```python
from build123d import *

# Parameters (mm, degrees)
SKETCH1_W           = 200
SKETCH1_H           = 200
BOSS_EXTRUDE1_DEPTH = 5
SKETCH3_R           = 2.5
CUT_EXTRUDE2_DEPTH  = 5
CUT_EXTRUDE4_DEPTH  = 200
CHAMFER1_SIZE       = 50
SKETCH5_R           = 2.5
CUT_EXTRUDE5_DEPTH  = 10


with BuildPart() as part:
    # Sketch1 → Boss-Extrude1 (new body)
    with BuildSketch(Plane(origin=(0, 0, 0), x_dir=(1, 0, 0), z_dir=(0, 1, 0))):
        with Locations((100, 100)):
            Rectangle(SKETCH1_W, SKETCH1_H)
    extrude(amount=BOSS_EXTRUDE1_DEPTH)

    # Sketch3 → Cut-Extrude2 (cut)
    with BuildSketch(Plane(origin=(0, 5, 0), x_dir=(1, 0, 0), z_dir=(0, 1, 0))):
        with Locations(Location((180, 62.426406871, 0), (0, 0, 270))):
            Circle(SKETCH3_R)
        with Locations(Location((90.710678119, 48.284271247, 0), (0, 0, 90))):
            Circle(SKETCH3_R)
        with Locations(Location((109.289321881, 48.284271247, 0), (0, 0, 270))):
            Circle(SKETCH3_R)
        with Locations(Location((62.426406871, 20, 0), (0, 0, 90))):
            Circle(SKETCH3_R)
        with Locations(Location((137.573593129, 20, 0), (0, 0, 270))):
            Circle(SKETCH3_R)
        with Locations(Location((20, 62.426406871, 0), (0, 0, 270))):
            Circle(SKETCH3_R)
        with Locations(Location((48.284271247, 90.710678119, 0), (0, 0, 270))):
            Circle(SKETCH3_R)
        with Locations(Location((20, 137.573593129, 0), (0, 0, 90))):
            Circle(SKETCH3_R)
        with Locations(Location((48.284271247, 109.289321881, 0), (0, 0, 90))):
            Circle(SKETCH3_R)
        with Locations(Location((62.426406871, 180, 0), (0, 0, 270))):
            Circle(SKETCH3_R)
        with Locations(Location((90.710678119, 151.715728753, 0), (0, 0, 270))):
            Circle(SKETCH3_R)
        with Locations(Location((109.289321881, 151.715728753, 0), (0, 0, 90))):
            Circle(SKETCH3_R)
        with Locations(Location((137.573593129, 180, 0), (0, 0, 90))):
            Circle(SKETCH3_R)
        with Locations(Location((180, 137.573593129, 0), (0, 0, 270))):
            Circle(SKETCH3_R)
        with Locations(Location((151.715728753, 109.289321881, 0), (0, 0, 270))):
            Circle(SKETCH3_R)
        with Locations(Location((151.715728753, 90.710678119, 0), (0, 0, 90))):
            Circle(SKETCH3_R)
    extrude(amount=-CUT_EXTRUDE2_DEPTH, mode=Mode.SUBTRACT)

    # Sketch4 → Cut-Extrude4 (cut)
    with BuildSketch(Plane(origin=(0, 5, 0), x_dir=(1, 0, 0), z_dir=(0, 1, 0))):
        Polygon((114.142135624, 121.213203436), (121.213203436, 114.142135624), (124.748737342, 117.67766953), (117.67766953, 124.748737342), align=None)
        Polygon((121.213203436, 85.857864376), (114.142135624, 78.786796564), (117.67766953, 75.251262658), (124.748737342, 82.32233047), align=None)
        Polygon((82.32233047, 75.251262658), (85.857864376, 78.786796564), (78.786796564, 85.857864376), (75.251262658, 82.32233047), align=None)
        Polygon((75.251262658, 117.67766953), (78.786796564, 114.142135624), (85.857864376, 121.213203436), (82.32233047, 124.748737342), align=None)
    extrude(amount=-CUT_EXTRUDE4_DEPTH, mode=Mode.SUBTRACT)

    # Chamfer1
    chamfer1_edges = [part.edges().sort_by_distance(p)[0] for p in [
        (0, 2.5, -200),
        (200, 2.5, -200),
        (200, 2.5, 0),
        (0, 2.5, 0),
    ]]
    chamfer(chamfer1_edges, length=CHAMFER1_SIZE)

    # Sketch5 → Cut-Extrude5 (cut)
    with BuildSketch(Plane(origin=(0, 5, 0), x_dir=(1, 0, 0), z_dir=(0, 1, 0))):
        with Locations(Location((41.213203436, 41.213203436, 0), (0, 0, 270))):
            Circle(SKETCH5_R)
        with Locations(Location((62.426406871, 137.573593129, 0), (0, 0, 270))):
            Circle(SKETCH5_R)
        with Locations(Location((41.213203436, 158.786796564, 0), (0, 0, 270))):
            Circle(SKETCH5_R)
        with Locations(Location((137.573593129, 137.573593129, 0), (0, 0, 270))):
            Circle(SKETCH5_R)
        with Locations(Location((158.786796564, 158.786796564, 0), (0, 0, 270))):
            Circle(SKETCH5_R)
        with Locations(Location((137.573593129, 62.426406871, 0), (0, 0, 270))):
            Circle(SKETCH5_R)
        with Locations(Location((158.786796564, 41.213203436, 0), (0, 0, 270))):
            Circle(SKETCH5_R)
        with Locations(Location((62.426406871, 62.426406871, 0), (0, 0, 270))):
            Circle(SKETCH5_R)
    extrude(amount=-CUT_EXTRUDE5_DEPTH, mode=Mode.SUBTRACT)


solid = part.part
```
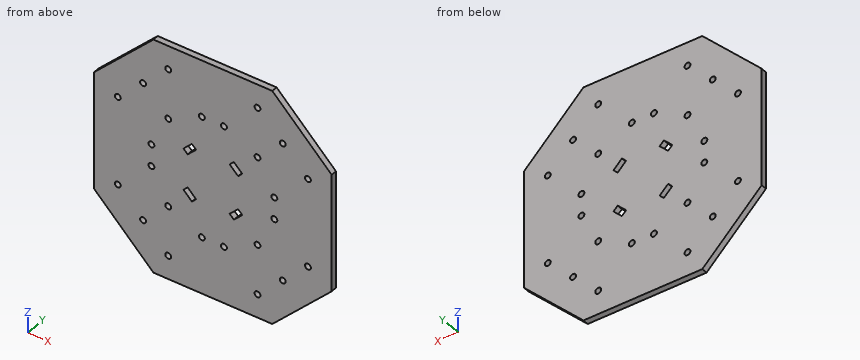
Here's how the part is built. I have some questions about the finished solid (model axes, mm). Round coordinates to 2 decimals unless told otherwise and drop trailing zeros. Write each loop counter-clockwise with the first axis right and the second up, starting at its lowest first coordinate (ties: lowest second). Pieces come first, ordered by that corner, then holes.
Q1. Please list where these lines run through material, in increasing order: probe 1 along Z at (x, y) = (19.5, 2.4); probe 2 along X at (y, z) = (3.85, -115.5); probe 3 along Z at (x, y) = (180, 1.65).
Q2. If we section it at C-C on y = 2.45: Give the number of separate pieces and of enclosed holes in the cut face, plus the area to 3 significant figures.
Q3. If we section it at B-B on z = -180: Write out the boundary of the cut face in (x, y), plus the area to 3 significant figures.
Q4. Will this pin go through, and if not, where does the flat tip stop? P1, Ø2, axis at x = 21, y = 2.5, coming from the +Z side.
Q5. If we section it at A-A on x = 20: Write out the boundary of the cut face in (y, z).
Answer below:
1. probe 1: z = -169.5 to -140.02, -135.12 to -64.88, -59.98 to -30.5
1. probe 2: x = 0 to 77.43, 80.14 to 119.86, 122.57 to 200
1. probe 3: z = -170 to -140.07, -135.07 to -64.93, -59.93 to -30
2. separate pieces: 1
2. enclosed holes: 28
2. area: 34,300 mm2
3. outline: (30, 0) - (59.93, 0) - (59.93, 5) - (30, 5) - close; (64.93, 0) - (135.07, 0) - (135.07, 5) - (64.93, 5) - close; (140.07, 0) - (170, 0) - (170, 5) - (140.07, 5) - close
3. area: 650 mm2
4. P1: stops at z = -28
5. outline: (0, -170) - (5, -170) - (5, -140.07) - (0, -140.07) - close; (0, -135.07) - (5, -135.07) - (5, -64.93) - (0, -64.93) - close; (0, -59.93) - (5, -59.93) - (5, -30) - (0, -30) - close
